Autodesk Inventor part; units mm, degrees
ref_plane "body_screw_XY" through (0, -6, 4) normal (0, 0, 1) x (1, 0, 0)
ref_plane "body_screw_YZ" through (0, -6, 4) normal (1, 0, 0) x (0, 1, 0)
ref_plane "body_screw_ZX" through (0, -6, 4) normal (0, 1, 0) x (0, 0, 1)
sketch "Sketch_1" plane through (0, 0, 0) normal (0, 0, 1) x (1, 0, 0)
  line L0 (4, 0) -> (-4, 0)
  line L1 (-4, 9.5) -> (-4, 3.5)
  line L2 (-4, 3.5) -> (-3.5, 3)
  line L3 (-3.5, 3) -> (3.5, 3)
  line L4 (3.5, 3) -> (4, 3.5)
  line L5 (4, 3.5) -> (4, 9.5)
  line L6 (4, 9.5) -> (3.5, 10)
  line L7 (3.5, 10) -> (-3.5, 10)
  line L8 (-3.5, 10) -> (-4, 9.5)
revolve "Revolution1" add sketch "Sketch_1" angle 360 about axis through (4, 0, 0) along (1, 0, 0)
sketch "Sketch_2" plane through (0, 0, 0) normal (1, 0, 0) x (0, 1, 0)
  line L0 (-10, 0.5) -> (-10, -0.5)
  line L1 (-10, -0.5) -> (6.25, -0.5)
  line L2 (6.25, -0.5) -> (6.25, 0.5)
  line L3 (6.25, 0.5) -> (-10, 0.5)
extrude "Extrusion1" cut sketch "Sketch_2" along normal mid plane 8
sketch "Sketch_3" plane through (0, 0, 0) normal (1, 0, 0) x (0, 1, 0)
  line L0 (-6, 10) -> (-6, 0)
  line L1 (-6, 0) -> (-7.7, 0)
  line L2 (-7.7, 0) -> (-7.7, 4)
  line L3 (-7.7, 4) -> (-9, 4)
  line L4 (-9, 4) -> (-9, 10)
  line L5 (-9, 10) -> (-6, 10)
  line L6 (-6, 10) -> (-6, 0)
revolve "Revolution2" cut sketch "Sketch_3" angle 360 about axis through (0, -6, 10) along (0, 0, 1)
sketch "Sketch4" plane through (-3.5, -2.958, -0.5) normal (0, 0, 1) x (1, 0, 0)
  point P0 (3.5, -3.042)
hole "Hole1" at (0, -6, -0.5) direction (0, 0, -1) diameter 2.459 depth 9 countersink diameter 3 countersink angle 90
sketch "Sketch_7" plane through (0, 0, -6) normal (0, 0, 1) x (1, 0, 0)
  line L0 (4, 0) -> (-4, 0)
  line L1 (-4, 0) -> (-4, 1.5)
  line L2 (-4, 1.5) -> (-3.7295, 1.2295)
  line L3 (-3.7295, 1.2295) -> (3.7295, 1.2295)
  line L4 (3.7295, 1.2295) -> (4, 1.5)
  line L5 (4, 1.5) -> (4, 0)
  line L6 (4, 0) -> (-4, 0)
revolve "Revolution3" cut sketch "Sketch_7" angle 360 about axis through (4, 0, -6) along (1, 0, 0)
thread "Thread1"
sketch "Sketch_8" plane through (0, 0, 6) normal (0, 0, 1) x (1, 0, 0)
  line L0 (4, 0) -> (-4, 0)
  line L1 (-4, 0) -> (-4, 1.5)
  line L2 (-4, 1.5) -> (-3.7295, 1.2295)
  line L3 (-3.7295, 1.2295) -> (3.7295, 1.2295)
  line L4 (3.7295, 1.2295) -> (4, 1.5)
  line L5 (4, 1.5) -> (4, 0)
  line L6 (4, 0) -> (-4, 0)
revolve "Revolution4" cut sketch "Sketch_8" angle 360 about axis through (4, 0, 6) along (1, 0, 0)
thread "Thread2"
ref_plane "body_screw_XY" through (0, -6, 4) normal (0, 0, 1) x (1, 0, 0)
ref_plane "body_screw_YZ" through (0, -6, 4) normal (1, 0, 0) x (0, 1, 0)
ref_plane "body_screw_ZX" through (0, -6, 4) normal (0, 1, 0) x (0, 0, 1)
properties part number "SCSW6-8b" material "鋼、炭素鋼"
The listing builds one solid part. Answer for the finished solid, in the listing's coordinates (mm). A direction names the side the tool comes from. Coordinates: 2 decimals unless noted, no trailing zeros. Write each loop counter-clockwise with the first axis right and the second up, starting at its lowest first coordinate (ties: lowest second). Pieces come first, ordered by that corner, then holes. Notation, with made-up numbers: (40, 67) -> (57, 67) arc R15 ccw to (57, 87) -> close; hole circle Ø3 at (-8.75, -26). An arc over 180 degrees is marked (long way). Write each question's results on one line, items separated by ' | '. Start each with the question number.
1) Straight lines are drawn through the part: probe 1 along Z at (x, y) = (0.75, 0); probe 2 along X at (y, z) = (-6, -6.5); probe 3 along X at (y, z) = (-6, 2.85). For each, find the intervals that lie inside material, in ascending order.
2) For a pull along Z with two mould halves and no side action, classify faces 6 (the cylindrical face through (0, 0, -3)), 7 (the flat face through (-4, 0, -4)) as +Z half, -Z half, draft (parallel to the pull), parting line (faces both ways), or undercut.
3) A cutting plane is placed at B-B (x = 0). Determine the outline of the cut face in (y, z).
4) A cutting plane is placed at A-A (y = 0). Count the separate pieces of the cut face and the enclosed holes in it, then the cut area to 3 significant figures.
5) A tool of negligible diameter and unlimited length cuts with its end or side. For faces 1 (the cylindrical face through (-1.03, -4.65, 2.27)), 2 (the conical face through (3.64, -0.06, -3.14)), 3 (the conical face through (-3.64, -0.06, 3.14)), 4 (the flat face through (0, 6.25, 0)), 5 (the cylindrical face through (0, 0, 3)), from which of +Z, -Z, +X, -X, +Y, -Y can it reach the whole face along a straight path? Write none if from no direction.
6) Flat-ended cylindrical pins translate along their axes: pin 1 Ø2.5 at (x, y) = (-1.5, 4.5) entering from +Z; pin 2 Ø1.5 at (x, y) = (-2, -6.5) entering from -Z; pin 3 Ø1 at (x, y) = (-1, 5) entering from -Z; pin 4 Ø1.5 at (x, y) = (0, -6) entering from -Z. Find the tip coordinate at first contact, or state that the pin passes through.
Values follow:
1) probe 1: -10 to -7.23, -4.77 to -3, 3 to 4.77, 7.23 to 10 | probe 2: -4 to -1.23, 1.23 to 4 | probe 3: -4 to -1.7, 1.7 to 4
2) face 6: undercut | face 7: draft
3) outline: (-9.99, -0.5) arc R10 ccw to (-7.23, -6.91) -> (-7.23, -0.77) -> (-7.5, -0.5) -> close; (-9.99, 0.5) -> (-7.7, 0.5) -> (-7.7, 4) -> (-9, 4) -> (-9, 4.36) arc R10 ccw to start; (-4.77, -8.79) arc R10 ccw (long way) to (-3, 9.54) -> (-3, 4) -> (-4.3, 4) -> (-4.3, 0.5) -> (-2.96, 0.5) arc R3 cw to (2.96, 0.5) -> (6.25, 0.5) -> (6.25, -0.5) -> (2.96, -0.5) arc R3 cw to (-2.96, -0.5) -> (-4.5, -0.5) -> (-4.77, -0.77) -> close; hole circle Ø2.46 at (0, -6); hole circle Ø2.46 at (0, 6)
4) separate pieces: 4 | enclosed holes: 0 | area: 71.4 mm²
5) face 1: +Z | face 2: +X | face 3: -X | face 4: +X, -X, -Y | face 5: +X, -X
6) pin 1: z = 9.46 | pin 2: z = -8.18 | pin 3: z = -8.93 | pin 4: through
